Job drawing, mm, ordinate dimensions from the low corner. One solid piece. A direction names the side the tool comes from. Round coordinates to 2 decimals unless told otherwise and drop trailing zeros. Loops run counter-clockwise (first coordinate to the right, second up) from the corner with the lowest first, then second, coordinate; pieces in that order, holes last. Notation, with made-up numbers: M -40,-26 L 11,-26 A7 ccw 11,-13 Z; hole C 54.25,35.5 d3. An arc over 180 degrees is marked long. One line per item, written item: value.
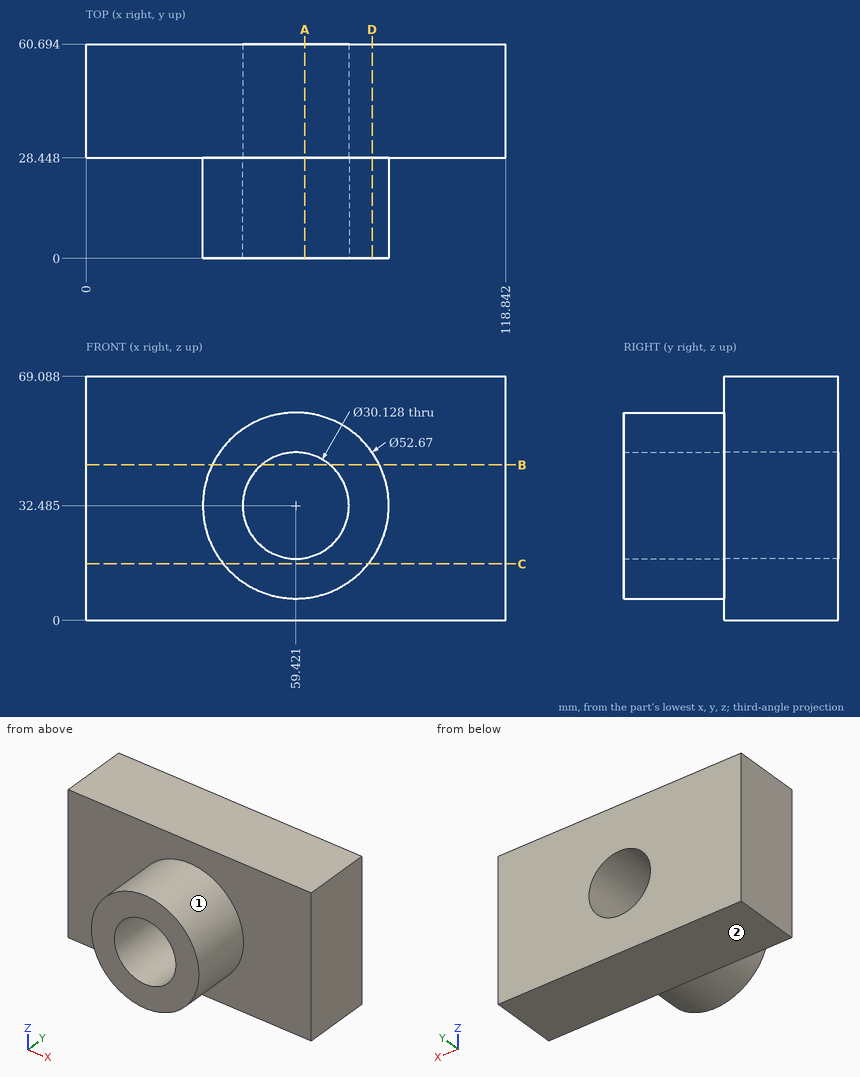
Item 1: Slice it at B-B, the plane z = 44. Give the cut face in (x, y) (1 decimal), and give its area (3 significant figures).
Check values:
outline: M 0,28.4 L 35.7,28.4 L 35.7,0 L 49.7,0 L 49.7,60.7 L 0,60.7 Z; M 69.1,0 L 83.1,0 L 83.1,28.4 L 118.8,28.4 L 118.8,60.7 L 69.1,60.7 Z
area: 4,000 mm2
Item 2: Slice it at C-C, the plane z = 16. Give the cut face in (x, y).
Check values:
outline: M 0,28.45 L 38.88,28.45 L 38.88,0 L 79.96,0 L 79.96,28.45 L 118.84,28.45 L 118.84,60.69 L 0,60.69 Z
Item 3: Wall check: line 1 along Y through (x, z) = (102, 55); line 2 along X through (y, z) = (49, 36); line 3 along X through (y, z) = (48.5, 46) (1 decimal). Give the ranges that are in metal, low to high.
Check values:
line 1: y = 28.45 to 60.69
line 2: x = 0 to 44.77, 74.07 to 118.84
line 3: x = 0 to 52.8, 66.1 to 118.8
Item 4: Slice it at D-D, the plane x = 81. Give the cut face in (y, z).
Check values:
outline: M 0,17.39 L 28.45,17.39 L 28.45,0 L 60.69,0 L 60.69,69.09 L 28.45,69.09 L 28.45,47.58 L 0,47.58 Z
Item 5: Slice it at A-A, the plane x = 62. Give the cut face in (y, z).
Check values:
outline: M 0,6.28 L 28.45,6.28 L 28.45,0 L 60.69,0 L 60.69,17.64 L 0,17.64 Z; M 0,47.33 L 60.69,47.33 L 60.69,69.09 L 28.45,69.09 L 28.45,58.69 L 0,58.69 Z
Item 6: Drop flat-ended pins along their axis: P1, Ø2, axis at y = 8.5, z = 36, coming from the +X side; P2, Ø12, axis at x = 36.5, z = 57.5, coming from the -Y side; P3, Ø18, axis at x = 59.42, z = 32.48, coming from the +Y side; P4, Ø1.5, axis at x = 37.5, y = 6.5, coming from the +Z side. Give the stop position or say it passes through.
Check values:
P1: stops at x = 85.64
P2: stops at y = 28.45
P3: passes through
P4: stops at z = 48.15
Item 7: Which spindle directions (+Z, -Z, +X, -X, +Y, -Y) get a long thin tool onto all of the face, cutting with end or side? Do the marked faces 1 and 2. Say none if no direction does.
Check values:
face 1: -Y
face 2: -Z, +X, -X, +Y, -Y
